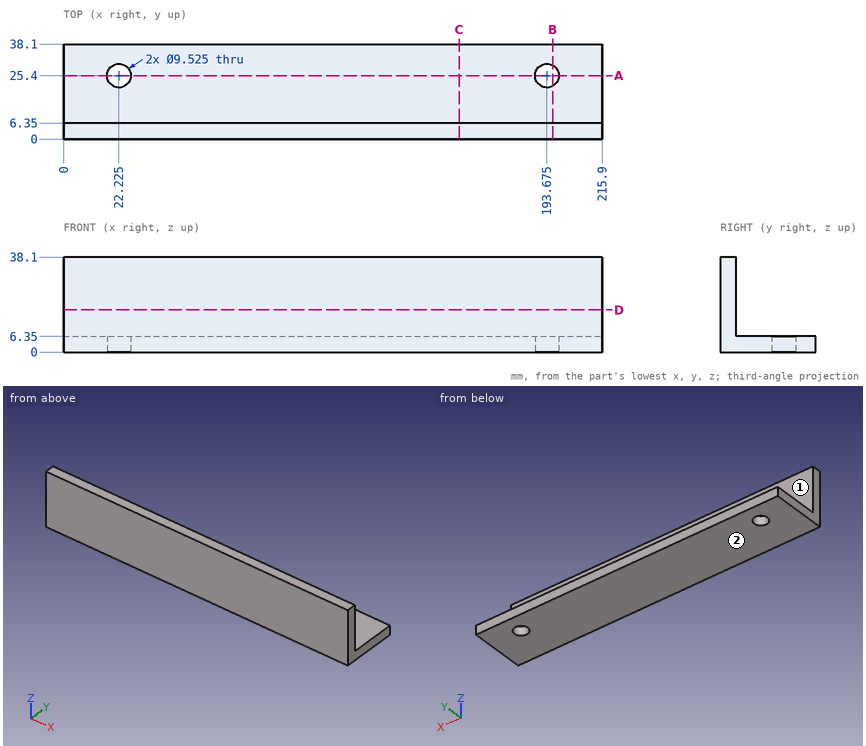
Job drawing, mm, ordinate dimensions from the low corner. One solid piece. A direction names the side the tool comes from. Give positions to 0.01 mm unless a question says otherwise; leave off trailing zeros. Loops run counter-clockwise (first coordinate to the right, second up) from the corner with the lowest first, then second, coordinate; pieces in that order, holes last.
Item 1: Slice it at C-C, the plane x = 158.5. List the corners of the cut face in (y, z).
Answers follow:
outline: (0, 0) - (38.1, 0) - (38.1, 6.35) - (6.35, 6.35) - (6.35, 38.1) - (0, 38.1) - close
Item 2: Which spindle directions (+Z, -Z, +X, -X, +Y, -Y) get a long thin tool onto all of the face, cutting with end or side? Do the marked faces 1 and 2. Say none if no direction does.
Answers follow:
face 1: +Z, +X, -X, +Y
face 2: -Z, +X, -X, +Y, -Y
Item 3: Slice it at A-A, the plane y = 25.4. List the corners of the cut face in (x, z), and give its area (3 significant figures).
Answers follow:
outline: (0, 0) - (17.46, 0) - (17.46, 6.35) - (0, 6.35) - close; (26.99, 0) - (188.91, 0) - (188.91, 6.35) - (26.99, 6.35) - close; (198.44, 0) - (215.9, 0) - (215.9, 6.35) - (198.44, 6.35) - close
area: 1,250 mm2
Item 4: Slice it at B-B, the plane x = 196. List the corners of the cut face in (y, z).
Answers follow:
outline: (0, 0) - (21.24, 0) - (21.24, 6.35) - (6.35, 6.35) - (6.35, 38.1) - (0, 38.1) - close; (29.56, 0) - (38.1, 0) - (38.1, 6.35) - (29.56, 6.35) - close
Item 5: Drill centre lines: line 1 (X direction, y = 25, z = 3); line 2 (Z direction, x = 181, y = 36). Where is each one in solid material? Low to high.
Answers follow:
line 1: x = 0 to 17.48, 26.97 to 188.93, 198.42 to 215.9
line 2: z = 0 to 6.35
Item 6: Flat gauge pins, fed straight in: pin 1 (3 mm diameter, centred on x = 68.5, y = 13, fed in from +Z); pin 2 (5.5 mm diameter, centred on x = 22.225, y = 25.4, fed in from -Z); pin 3 (16 mm diameter, centred on x = 105, z = 20.5, fed in from +Y). Where does each tip first touch, or does it go through?
Answers follow:
pin 1: stops at z = 6.35
pin 2: passes through
pin 3: stops at y = 6.35
Item 7: Slice it at D-D, the plane z = 17. List the corners of the cut face in (x, y), and give its area (3 significant figures).
Answers follow:
outline: (0, 0) - (215.9, 0) - (215.9, 6.35) - (0, 6.35) - close
area: 1,370 mm2
